from build123d import *

# Parameters (mm, degrees)
CYLINDER416_R     = 2.5
CYLINDER416_DEPTH = 10
CYLINDER418_R     = 21.5
CYLINDER418_DEPTH = 63
BOX001_W          = 5
BOX001_H          = 10
BOX001_DEPTH      = 10
CYLINDER417_R     = 5
CYLINDER417_DEPTH = 10


with BuildPart() as cylinder416:
    # Cylinder416 → Cylinder416 (new body)
    with BuildSketch(Plane(origin=(25, -4, 0), x_dir=(1, 0, 0), z_dir=(0, 0, 1))):
        Circle(CYLINDER416_R)
    extrude(amount=CYLINDER416_DEPTH)


with BuildPart() as fusion093:
    # Cylinder418 → Cylinder418 (new body)
    with BuildSketch(Plane.XY):
        Circle(CYLINDER418_R)
    extrude(amount=CYLINDER418_DEPTH)

    # Fusion093: union Cylinder416
    add(cylinder416.part)


with BuildPart() as cube001:
    # Box001 → Box001 (new body)
    with BuildSketch(Plane(origin=(20, -9, 0), x_dir=(1, 0, 0), z_dir=(0, 0, 1))):
        with Locations((2.5, 5)):
            Rectangle(BOX001_W, BOX001_H)
    extrude(amount=BOX001_DEPTH)


with BuildPart() as slider:
    # Cylinder417 → Cylinder417 (new body)
    with BuildSketch(Plane(origin=(25, -4, 0), x_dir=(1, 0, 0), z_dir=(0, 0, 1))):
        Circle(CYLINDER417_R)
    extrude(amount=CYLINDER417_DEPTH)

    # Fusion092: union Cube001
    add(cube001.part)

    # Cut236: cut Fusion093
    add(fusion093.part, mode=Mode.SUBTRACT)


with BuildPart() as slider_1:
    # Cut236 placement: moved
    add(slider.part.moved(Location((0, 0, 22))))


solid = slider_1.part
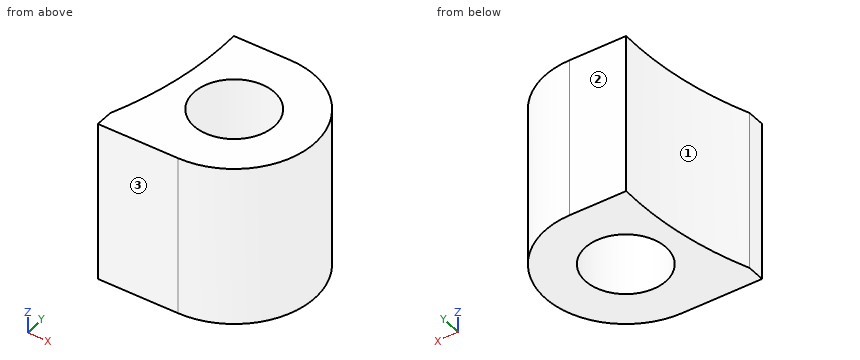
Could you check a few things on this model? Use its own coordinates, in mm. Face numbers are marked on the shaded views. Round coordinates to 2 decimals unless told otherwise and drop trailing zeros. Order: outer loops, then holes, each group sorted by start corner. A loop starts at its lowest first (then second) coordinate and runs counter-clockwise, first axis right, second up.
(1) If we mould it in two halves opening along Y, with no side actions, what happens to the marked faces 1, 2 and 3? For each: released by +Y, released by -Y, zero draft, split by the parting line, or undercut.
Response values:
face 1: undercut
face 2: released by +Y
face 3: released by -Y
(2) I'm going to push a flat-ended pin straight in: pin 1 (1 mm diameter, centred on x = 26.5, z = 24, fed in from -Y). Where does the tip first touch, or does it pass through?
Response values:
pin 1: stops at y = -8.9
(3) Imagine slicing it at D-D (x = 28). Write out the boundary of the cut face in (y, z), plus the area to 3 significant figures.
Response values:
outline: (-8, 22) - (0, 22) - (0, 32) - (-8, 32) - close
area: 80.0 mm2
(4) Imagine slicing it at B-B (z = 26). Write out the boundary of the cut face in (x, y).
Response values:
outline: (20, -9) - (25, -9) arc R5 ccw to (25, 1) - (21.48, 1) arc R21.5 cw to (20, -7.89) - close; hole circle Ø5 at (25, -4)
(5) Imagine slicing it at A-A (y = -4). Write out the boundary of the cut face in (x, z), plus the area to 3 significant figures.
Response values:
outline: (21.12, 22) - (22.5, 22) - (22.5, 32) - (21.12, 32) - close; (27.5, 22) - (30, 22) - (30, 32) - (27.5, 32) - close
area: 38.8 mm2
(6) Imagine slicing it at C-C (x = 25.75). Write out the boundary of the cut face in (y, z), plus the area to 3 significant figures.
Response values:
outline: (-8.94, 22) - (-6.38, 22) - (-6.38, 32) - (-8.94, 32) - close; (-1.62, 22) - (0.94, 22) - (0.94, 32) - (-1.62, 32) - close
area: 51.2 mm2
(7) Please list where these lines run through material, in increasing order: line 1 along Y through (x, z) = (25, 28.5); line 2 along X through (y, z) = (-4.25, 29.5); line 3 along Y through (x, z) = (27.25, 29.25).
Response values:
line 1: y = -9 to -6.5, -1.5 to 1
line 2: x = 21.08 to 22.51, 27.49 to 29.99
line 3: y = -8.47 to -5.09, -2.91 to 0.47
